```python
from build123d import *

# Parameters (mm, degrees)
F2_R     = 40
F3_R     = 5
F4_R     = 5
F5_R     = 4.25
F6_DEPTH = 10
F7_COUNT = 3


# Not quite as in the source:
# - a feature names something its author has since deleted; it is built from what else it names


with BuildPart() as f1:
    # F0 (on Right) → F1 (revolve)
    with BuildSketch(Plane.YZ):
        Polygon((115.0588170719, 135), (-104.9411829281, 135), (-104.9411829281, 62.5099688768), (-74.9411829281, 62.5099688768), (-24.9411829281, 37.5), (-10.9411829281, 37.5), (-10.9411829281, 20), (-0.9411829281, 20), (-0.9411829281, 37.5), (23.0588170719, 37.5), (65.0588170719, 58.5), (115.0588170719, 58.5), align=None)
    revolve(axis=Axis((0, 3.7167160804, 0), (0, -1, 0)))

    # F2
    f2_edges = [f1.edges().sort_by_distance(p)[0] for p in [
        (0, -104.941183, -135),
        (0, 115.058817, -135),
    ]]
    fillet(f2_edges, radius=F2_R)

    # F3
    f3_edges = [f1.edges().sort_by_distance(p)[0] for p in [
        (0, -104.941183, -62.509969),
    ]]
    fillet(f3_edges, radius=F3_R)

    # F4
    f4_edges = [f1.edges().sort_by_distance(p)[0] for p in [
        (0, 115.058817, -58.5),
    ]]
    fillet(f4_edges, radius=F4_R)

    # F5 (on face) → F6 (cut, through all)
    with BuildSketch(Plane.XZ.offset(10.9411829281)):
        with Locations((0, 29)):
            Circle(F5_R)
    f6 = extrude(amount=-F6_DEPTH, mode=Mode.SUBTRACT)

    # F7: F6 ×3 about axis
    f7_axis = Axis((0, 3.7167160804, 0), (0, -1, 0))
    for i in range(1, F7_COUNT):
        add(f6.rotate(f7_axis, i * 360 / F7_COUNT), mode=Mode.SUBTRACT)


solid = f1.part
```
CAD build for the part. Positions are in the model's coordinates, mm. A direction names the side the tool comes from. Round coordinates to 2 decimals unless told otherwise and drop trailing zeros. Loops run counter-clockwise (first coordinate to the right, second up) from the corner with the lowest first, then second, coordinate; pieces in that order, holes last. Notation, with made-up numbers: M -14.5,-36.5 L 11.5,-36.5 A25 ccw 11.5,-20.5 Z; hole C -35.75,73 d8. An arc over 180 degrees is marked long. Return JSON: item names as keys, results as strings. Group by question number.
(1) Saw through at D-D, the plane y = -88.5. List the corners of the cut face in (x, z), and give its area (3 significant figures).
(2) Tool access for faces 1 (the cylindrical face through (-37.18, -17.84, -4.88)), 2 (the cylindrical face through (-37.18, 11.23, -4.88)), 3 (the cylindrical face through (19.524, -5.871, -4.336)): list every direction of +Z, -Z, +X, -X, +Y, -Y with a clear straight run to the whole face (end or side of a thin tool).
(3) Drop flat-ended pins along their axis: P1, Ø12, axis at x = 29.5, z = -1.5, coming from the +Y side; P2, Ø8, axis at x = -62.5, y = 38, coming from the -Z side; P3, Ø1.5, axis at x = -74.5, z = -98.5, coming from the +Y side. Give the stop position or say it passes through.
(4) Saw through at C-C, the plane y = 37. List the corners of the cut face in (x, z).
(5) Wall check: probe 1 along X at (y, z) = (-19, 0); probe 2 along X at (y, z) = (-6.5, 0); probe 3 along Z at (x, y) = (0, -83). Give the ranges that are in metal, low to high. Write a range as [from, to].
(6) Saw through at B-B, the plane x = 0. Give the number of separate pieces and of enclosed holes in the cut face, and give its area (3 significant figures).
(7) Mould opens along Z. For faces 4 (the cylindrical face through (82.15, 4.08, -107.13)), 5 (the conical face through (37.9, 25.7, -8.4)), 6 (the flat face through (20, 115.059, -62)) say: +Z half, -Z half, draft (parallel to the pull), parting line (faces both ways), or undercut.
Answer list:
{
 "1": {"outline": "C 0,0 d254.65; hole C 0,0 d125.02", "area": "38,700 mm2"},
 "2": {"face 1": "-Y", "face 2": "+Y", "face 3": "+Y, -Y"},
 "3": {"P1": "y = -0.94", "P2": "z = -121.67", "P3": "y = 103.87"},
 "4": {"outline": "C 0,0 d270; hole C 0,0 d88.94"},
 "5": {"probe 1": "[-135, -37.5], [37.5, 135]", "probe 2": "[-135, -20], [20, 135]", "probe 3": "[-130.69, -62.51], [62.51, 130.69]"},
 "6": {"separate pieces": "3", "enclosed holes": "0", "area": "36,000 mm2"},
 "7": {"face 4": "parting line", "face 5": "undercut", "face 6": "draft"}
}
